Geometry check sheet. Reference: the model listing, model coordinates, mm. Face numbers are marked on the shaded views. A direction names the side the tool comes from. Coordinates: 2 decimals unless noted, no trailing zeros. Write each loop counter-clockwise with the first axis right and the second up, starting at its lowest first coordinate (ties: lowest second). Pieces come first, ordered by that corner, then holes.
from build123d import *

# Parameters (mm, degrees)
F2_R    = 1
F3_SIZE = 1


with BuildPart() as f1:
    # F0 (on Right) → F1 (revolve)
    with BuildSketch(Plane.YZ):
        Polygon((2.5, 27), (2.5, 0), (7.5, 0), (7.5, 30), (2.5, 30), (2.5, 45), (0, 45), (0, 27), align=None)
    revolve(axis=Axis((0, 0, 12.798217), (0, 0, -1)))

    # F2
    f2_edges = [f1.edges().sort_by_distance(p)[0] for p in [
        (0, -2.5, 45),
        (0, -2.5, 30),
        (0, -7.5, 30),
    ]]
    fillet(f2_edges, radius=F2_R)

    # F3
    f3_edges = [f1.edges().sort_by_distance(p)[0] for p in [
        (0, -7.5, 0),
    ]]
    chamfer(f3_edges, length=F3_SIZE)


solid = f1.part
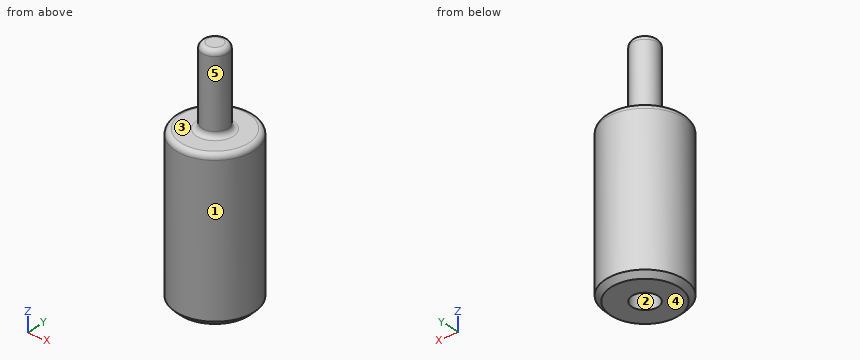
1. Sectioned sample at D-D, the plane z = 39.5. Record the boundary of the cut face in (x, y).
Computed values:
outline: circle Ø5 at (0, 0)
2. Draft check along Y on the marked faces 1, 2 and 3. Enter one of: released by +Y, released by -Y, zero draft, split by the parting line, or undercut.
Computed values:
face 1: split by the parting line
face 2: undercut
face 3: zero draft
3. Gauge pin test, flat ends, axial feed: pin 1 Ø6 at (x, y) = (-1.5, 3.5) entering from +Z; pin 2 Ø8 at (y, z) = (-3, 39) entering from +X; pin 3 Ø4 at (x, y) = (4, -6) entering from +Z; pin 4 Ø2.5 at (x, y) = (-0.5, -1) entering from -Z. Record the tip position at first contact, or that the pin passes through.
Computed values:
pin 1: stops at z = 45
pin 2: stops at x = 2.5
pin 3: stops at z = 30
pin 4: stops at z = 27
4. Thickness scan on line 1 along X through (y, z) = (0, 6.25); line 2 along X through (y, z) = (-3.75, 24.5); line 3 along X through (y, z) = (-2, 2). Record the ranges inside material, lowest first.
Computed values:
line 1: x = -7.5 to -2.5, 2.5 to 7.5
line 2: x = -6.5 to 6.5
line 3: x = -7.23 to -1.5, 1.5 to 7.23
5. Sectioned sample at A-A, the plane x = 0. Record the boundary of the cut face in (y, z).
Computed values:
outline: (-7.5, 1) - (-6.5, 0) - (-2.5, 0) - (-2.5, 27) - (2.5, 27) - (2.5, 0) - (6.5, 0) - (7.5, 1) - (7.5, 29) arc R1 ccw to (6.5, 30) - (3.5, 30) arc R1 cw to (2.5, 31) - (2.5, 44) arc R1 ccw to (1.5, 45) - (-1.5, 45) arc R1 ccw to (-2.5, 44) - (-2.5, 31) arc R1 cw to (-3.5, 30) - (-6.5, 30) arc R1 ccw to (-7.5, 29) - close
6. Access from +Z, -Z, +X, -X, +Y, -Y to the whole of each face (thin tool, end or side, straight path). Record for the marked faces 4 and 5.
Computed values:
face 4: -Z, +X, -X, +Y, -Y
face 5: +Z
7. Sectioned sample at B-B, the plane z = 11.5. Record the boundary of the cut face in (x, y), and give its area (3 significant figures).
Computed values:
outline: circle Ø15 at (0, 0); hole circle Ø5 at (0, 0)
area: 157 mm2
